Part model, mm, in its own coordinate system. A direction names the side the tool comes from. Coordinates: 2 decimals unless noted, no trailing zeros. Order: outer loops, then holes, each group sorted by start corner. A loop starts at its lowest first (then second) coordinate and runs counter-clockwise, first axis right, second up.
from build123d import *

# Parameters (mm, degrees)
SKETCH1_W               = 44
SKETCH1_H               = 277
SKETCH1_W_2             = 6
SKETCH1_H_2             = 9
SKETCH1_W_3             = 9.5
SKETCH1_H_3             = 6
BOSS_EXTRUDE1_DEPTH     = 6
CUT_EXTRUDE1_DEPTH      = 288.445647036
CUT_EXTRUDE1_DEPTH_BACK = 288.445647036
SKETCH2_R               = 2.75
CUT_EXTRUDE2_DEPTH      = 288.445647036
CUT_EXTRUDE2_DEPTH_BACK = 288.445647036
SKETCH3_R               = 1.6
SKETCH3_W               = 4
SKETCH3_H               = 4
CUT_EXTRUDE3_DEPTH      = 288.445647036
CUT_EXTRUDE3_DEPTH_BACK = 288.445647036
SKETCH4_R               = 2.5
CUT_EXTRUDE4_DEPTH      = 288.445647036
CUT_EXTRUDE4_DEPTH_BACK = 288.445647036
SKETCH5_R               = 1.6


with BuildPart() as part:
    # Sketch1 → Boss-Extrude1 (new body)
    with BuildSketch(Plane(origin=(0, 0, 0), x_dir=(1, 0, 0), z_dir=(0, 1, 0))):
        with Locations((22, 138.5)):
            Rectangle(SKETCH1_W, SKETCH1_H)
        with Locations((-3, 12)):
            Rectangle(SKETCH1_W_2, SKETCH1_H_2)
        with Locations((-3, 32)):
            Rectangle(SKETCH1_W_2, SKETCH1_H_2)
        with Locations((-3, 52)):
            Rectangle(SKETCH1_W_2, SKETCH1_H_2)
        with Locations((-3, 72)):
            Rectangle(SKETCH1_W_2, SKETCH1_H_2)
        with Locations((-3, 92)):
            Rectangle(SKETCH1_W_2, SKETCH1_H_2)
        with Locations((-3, 112)):
            Rectangle(SKETCH1_W_2, SKETCH1_H_2)
        with Locations((-3, 132)):
            Rectangle(SKETCH1_W_2, SKETCH1_H_2)
        with Locations((-3, 152)):
            Rectangle(SKETCH1_W_2, SKETCH1_H_2)
        with Locations((-3, 172)):
            Rectangle(SKETCH1_W_2, SKETCH1_H_2)
        with Locations((-3, 192)):
            Rectangle(SKETCH1_W_2, SKETCH1_H_2)
        with Locations((-3, 212)):
            Rectangle(SKETCH1_W_2, SKETCH1_H_2)
        with Locations((-3, 232)):
            Rectangle(SKETCH1_W_2, SKETCH1_H_2)
        with Locations((-3, 252)):
            Rectangle(SKETCH1_W_2, SKETCH1_H_2)
        with Locations((-3, 272)):
            Rectangle(SKETCH1_W_2, SKETCH1_H_2)
        with Locations((12, 280)):
            Rectangle(SKETCH1_W_3, SKETCH1_H_3)
        with Locations((32, 280)):
            Rectangle(SKETCH1_W_3, SKETCH1_H_3)
        with Locations((47, 272)):
            Rectangle(SKETCH1_W_2, SKETCH1_H_2)
        with Locations((47, 252)):
            Rectangle(SKETCH1_W_2, SKETCH1_H_2)
        with Locations((47, 232)):
            Rectangle(SKETCH1_W_2, SKETCH1_H_2)
        with Locations((47, 212)):
            Rectangle(SKETCH1_W_2, SKETCH1_H_2)
        with Locations((47, 192)):
            Rectangle(SKETCH1_W_2, SKETCH1_H_2)
        with Locations((47, 172)):
            Rectangle(SKETCH1_W_2, SKETCH1_H_2)
        with Locations((47, 152)):
            Rectangle(SKETCH1_W_2, SKETCH1_H_2)
        with Locations((47, 132)):
            Rectangle(SKETCH1_W_2, SKETCH1_H_2)
        with Locations((47, 112)):
            Rectangle(SKETCH1_W_2, SKETCH1_H_2)
        with Locations((47, 92)):
            Rectangle(SKETCH1_W_2, SKETCH1_H_2)
        with Locations((47, 72)):
            Rectangle(SKETCH1_W_2, SKETCH1_H_2)
        with Locations((47, 52)):
            Rectangle(SKETCH1_W_2, SKETCH1_H_2)
        with Locations((47, 32)):
            Rectangle(SKETCH1_W_2, SKETCH1_H_2)
        with Locations((47, 12)):
            Rectangle(SKETCH1_W_2, SKETCH1_H_2)
    extrude(amount=BOSS_EXTRUDE1_DEPTH)

    # Sketch2 → Cut-Extrude1 (cut, two sides: drawn at the far end of the back side and taken through both)
    with BuildSketch(Plane(origin=(0, 6, 0), x_dir=(1, 0, 0), z_dir=(0, 1, 0)).offset(-CUT_EXTRUDE1_DEPTH_BACK)):
        with Locations(Location((6, 267, 0), (0, 0, 270))):
            Circle(SKETCH2_R)
        with Locations(Location((38, 267, 0), (0, 0, 270))):
            Circle(SKETCH2_R)
    extrude(amount=CUT_EXTRUDE1_DEPTH + CUT_EXTRUDE1_DEPTH_BACK, mode=Mode.SUBTRACT)

    # Sketch3 → Cut-Extrude2 (cut, two sides: drawn at the far end of the back side and taken through both)
    with BuildSketch(Plane(origin=(0, 6, 0), x_dir=(1, 0, 0), z_dir=(0, 1, 0)).offset(-CUT_EXTRUDE2_DEPTH_BACK)):
        with Locations(Location((16, 237, 0), (0, 0, 270))):
            Circle(SKETCH3_R)
        with Locations(Location((28, 237, 0), (0, 0, 270))):
            Circle(SKETCH3_R)
        with Locations((16, 242)):
            Rectangle(SKETCH3_W, SKETCH3_H)
        with Locations((16, 232)):
            Rectangle(SKETCH3_W, SKETCH3_H)
        with Locations((28, 242)):
            Rectangle(SKETCH3_W, SKETCH3_H)
        with Locations((28, 232)):
            Rectangle(SKETCH3_W, SKETCH3_H)
    extrude(amount=CUT_EXTRUDE2_DEPTH + CUT_EXTRUDE2_DEPTH_BACK, mode=Mode.SUBTRACT)

    # Sketch4 → Cut-Extrude3 (cut, two sides: drawn at the far end of the back side and taken through both)
    with BuildSketch(Plane(origin=(0, 6, 0), x_dir=(1, 0, 0), z_dir=(0, 1, 0)).offset(-CUT_EXTRUDE3_DEPTH_BACK)):
        with Locations(Location((33, 39, 0), (0, 0, 270))):
            Circle(SKETCH4_R)
        with Locations(Location((11, 39, 0), (0, 0, 270))):
            Circle(SKETCH4_R)
    extrude(amount=CUT_EXTRUDE3_DEPTH + CUT_EXTRUDE3_DEPTH_BACK, mode=Mode.SUBTRACT)

    # Sketch5 → Cut-Extrude4 (cut, two sides: drawn at the far end of the back side and taken through both)
    with BuildSketch(Plane(origin=(0, 6, 0), x_dir=(1, 0, 0), z_dir=(0, 1, 0)).offset(-CUT_EXTRUDE4_DEPTH_BACK)):
        with Locations(Location((-3, 12, 0), (0, 0, 270))):
            Circle(SKETCH5_R)
        with Locations(Location((47, 12, 0), (0, 0, 270))):
            Circle(SKETCH5_R)
        with Locations(Location((47, 52, 0), (0, 0, 270))):
            Circle(SKETCH5_R)
        with Locations(Location((47, 92, 0), (0, 0, 270))):
            Circle(SKETCH5_R)
        with Locations(Location((47, 132, 0), (0, 0, 270))):
            Circle(SKETCH5_R)
        with Locations(Location((47, 172, 0), (0, 0, 270))):
            Circle(SKETCH5_R)
        with Locations(Location((47, 212, 0), (0, 0, 270))):
            Circle(SKETCH5_R)
        with Locations(Location((-3, 52, 0), (0, 0, 270))):
            Circle(SKETCH5_R)
        with Locations(Location((-3, 92, 0), (0, 0, 270))):
            Circle(SKETCH5_R)
        with Locations(Location((-3, 132, 0), (0, 0, 270))):
            Circle(SKETCH5_R)
        with Locations(Location((-3, 172, 0), (0, 0, 270))):
            Circle(SKETCH5_R)
        with Locations(Location((-3, 212, 0), (0, 0, 270))):
            Circle(SKETCH5_R)
        with Locations(Location((32, 280, 0), (0, 0, 270))):
            Circle(SKETCH5_R)
        with Locations(Location((12, 280, 0), (0, 0, 270))):
            Circle(SKETCH5_R)
    extrude(amount=CUT_EXTRUDE4_DEPTH + CUT_EXTRUDE4_DEPTH_BACK, mode=Mode.SUBTRACT)


solid = part.part
Q1. Which spindle directions (+Z, -Z, +X, -X, +Y, -Y) get a long thin tool onto all of the face, cutting with end or side? Do faces 4 (the face through (47, 3, -236.5)), 5 (the face through (-3, 3, -16.5)), 6 (the face through (4, 3, -277)). Say none if no direction does.
Results list:
face 4: +X, +Y, -Y
face 5: -X, +Y, -Y
face 6: -Z, -X, +Y, -Y
Q2. Pin check, flat tips, straight feed: pin 1 Ø2.5 at (x, z) = (47, -132) entering from +Y; pin 2 Ø1.8 at (x, y) = (46.5, 2.5) entering from +Z; pin 3 Ø3 at (x, y) = (-3.5, 4.5) entering from -Z. Stop position of each tip, or through.
Results list:
pin 1: passes through
pin 2: stops at z = -7.5
pin 3: stops at z = -276.5
Q3. Wall check: line 1 along X through (y, z) = (2.65, -52); line 2 along X through (y, z) = (1.95, -267); line 3 along Z through (x, y) = (15.5, 4). Give the ranges that are in metal, low to high.
Results list:
line 1: x = -6 to -4.6, -1.4 to 45.4, 48.6 to 50
line 2: x = 0 to 3.25, 8.75 to 35.25, 40.75 to 44
line 3: z = -283 to -244, -240 to -238.52, -235.48 to -234, -230 to 0
Q4. Cut at B-B on y = 2.4. Count the separate pieces of the cut face and the enclosed holes in it, and give its area (3 significant figures).
Results list:
separate pieces: 1
enclosed holes: 24
area: 13,500 mm2
Q5. Mould opens along Z. For faces 1 (the face through (-3, 3, -276.5)), 2 (the face through (-6, 3, -32)), 3 (the face through (38.83, 2.96, -264.38)) say: pulls with the +Z half, pulls with the -Z half, needs draft (parallel to the pull), parting line crosses it, or undercut.
Results list:
face 1: pulls with the -Z half
face 2: needs draft
face 3: undercut
Q6. Cut at A-A on z = -219.5. Write the cut outline in (x, y), and give its area (3 significant figures).
Results list:
outline: (0, 0) - (44, 0) - (44, 6) - (0, 6) - close
area: 264 mm2
